Work out the finished part from the listing and answer in its coordinate system (mm). Face numbers are marked on the shaded views. Give positions to 0.01 mm unless a question says otherwise; leave off trailing zeros. Write each loop counter-clockwise with the first axis right and the second up, starting at its lowest first coordinate (ties: lowest second). Pieces come first, ordered by that corner, then holes. Notation, with made-up numbers: (18.5, -11.5) -> (30.5, -11.5) arc R20 ccw to (30.5, 26.5) -> close; hole circle Ø4 at (34.25, 88). An arc over 180 degrees is marked (long way). Use a Markdown table: item, result. Add a question column.
Q1. For a pull along X with two mould halves and no side action, classify the marked faces 1, 2, 3 and 4 as pulls with the +X half, pulls with the -X half, needs draft (parallel to the pull), parting line crosses it, or undercut.
Q2. Section B-B, the plane x = -8 is taken. Give the vertices of the cut face in (y, z).
Q3. Consider line 1 (Z direction, x = -15.5, y = -14.5); line 2 (Z direction, x = 14, y = -6); line 3 (X direction, y = -5.25, z = -12.5). Determine where each line is inside the solid, lowest interval first.
Q4. Section C-C, the plane z = 7 is taken. Give the vertices of the cut face in (x, y), plus the area to 3 significant figures.
Q5. Each of these flat-tipped pins is pushed along its axis until it touches: pin 1 Ø5 at (x, y) = (-0.5, -10) entering from -Z; pin 2 Ø6 at (x, y) = (-16, -16.5) entering from -Z; pin 3 Ø1.5 at (y, z) = (-12, 5) entering from -X; pin 4 Ø8 at (x, y) = (12.5, -13) entering from +Z. Where does it stop, or does it pass through?
Q6. Section A-A, the plane x = -17 is taken. Give the vertices of the cut face in (y, z).
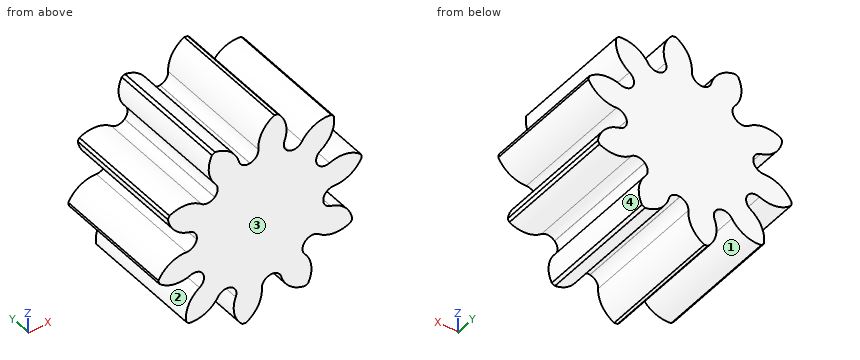
from build123d import *

# Parameters (mm, degrees)
F1_DEPTH = 25


with BuildPart() as f1:
    # F0 (on Front) → F1 (new body)
    with BuildSketch(Plane.XZ):
        with BuildLine():
            ThreePointArc((-0.348561, 15.07019), (-0.783748, 13.691524), (-2.03445, 12.966366))
            ThreePointArc((-2.03445, 12.966366), (-2.044108, 12.964847), (-2.053766, 12.96332))
            ThreePointArc((-2.053766, 12.96332), (-2.063307, 12.961805), (-2.072847, 12.960283))
            ThreePointArc((-2.072847, 12.960283), (-3.48649, 13.263394), (-4.326471, 14.440126))
            ThreePointArc((-4.326471, 14.440126), (-6.102339, 17.389838), (-9.209645, 18.872796))
            ThreePointArc((-9.209645, 18.872796), (-9.534613, 18.710723), (-9.856731, 18.543054))
            ThreePointArc((-9.856731, 18.543054), (-10.48276, 15.157493), (-9.140028, 11.987161))
            ThreePointArc((-9.140028, 11.987161), (-8.681741, 10.616), (-9.267343, 9.294191))
            ThreePointArc((-9.267343, 9.294191), (-9.274264, 9.287285), (-9.28118, 9.280373))
            ThreePointArc((-9.28118, 9.280373), (-9.288008, 9.273539), (-9.294832, 9.2667))
            ThreePointArc((-9.294832, 9.2667), (-10.616657, 8.681004), (-11.987881, 9.139271))
            ThreePointArc((-11.987881, 9.139271), (-15.158386, 10.48181), (-18.54391, 9.85512))
            ThreePointArc((-18.54391, 9.85512), (-18.711551, 9.532987), (-18.873597, 9.208005))
            ThreePointArc((-18.873597, 9.208005), (-17.390082, 6.101058), (-14.440314, 4.325444))
            ThreePointArc((-14.440314, 4.325444), (-13.263604, 3.485525), (-12.960426, 2.071951))
            ThreePointArc((-12.960426, 2.071951), (-12.961966, 2.062295), (-12.963499, 2.052639))
            ThreePointArc((-12.963499, 2.052639), (-12.965006, 2.043097), (-12.966506, 2.033553))
            ThreePointArc((-12.966506, 2.033553), (-13.691622, 0.782765), (-15.070328, 0.347526))
            ThreePointArc((-15.070328, 0.347526), (-18.424445, -0.429914), (-20.795033, -2.926878))
            ThreePointArc((-20.795033, -2.926878), (-20.741312, -3.286025), (-20.68139, -3.64419))
            ThreePointArc((-20.68139, -3.64419), (-17.654983, -5.285774), (-14.224891, -4.988446))
            ThreePointArc((-14.224891, -4.988446), (-12.779221, -4.976302), (-11.703067, -5.941704))
            ThreePointArc((-11.703067, -5.941704), (-11.698638, -5.95042), (-11.694202, -5.959133))
            ThreePointArc((-11.694202, -5.959133), (-11.689812, -5.96774), (-11.685416, -5.976342))
            ThreePointArc((-11.685416, -5.976342), (-11.536853, -7.414464), (-12.396423, -8.576962))
            ThreePointArc((-12.396423, -8.576962), (-14.652992, -11.177425), (-15.103159, -14.590907))
            ThreePointArc((-15.103159, -14.590907), (-14.848597, -14.849888), (-14.589595, -15.104427))
            ThreePointArc((-14.589595, -15.104427), (-11.176282, -14.65362), (-8.576044, -12.396919))
            ThreePointArc((-8.576044, -12.396919), (-7.41361, -11.537351), (-5.975534, -11.68583))
            ThreePointArc((-5.975534, -11.68583), (-5.966827, -11.690278), (-5.958117, -11.69472))
            ThreePointArc((-5.958117, -11.69472), (-5.949507, -11.699102), (-5.940895, -11.703478))
            ThreePointArc((-5.940895, -11.703478), (-4.975398, -12.779619), (-4.987505, -14.225343))
            ThreePointArc((-4.987505, -14.225343), (-5.284594, -17.65554), (-3.642392, -20.681706))
            ThreePointArc((-3.642392, -20.681706), (-3.284223, -20.741598), (-2.925071, -20.795287))
            ThreePointArc((-2.925071, -20.795287), (-0.42862, -18.424281), (0.348561, -15.07019))
            ThreePointArc((0.348561, -15.07019), (0.783748, -13.691524), (2.03445, -12.966366))
            ThreePointArc((2.03445, -12.966366), (2.044108, -12.964847), (2.053766, -12.96332))
            ThreePointArc((2.053766, -12.96332), (2.063307, -12.961805), (2.072847, -12.960283))
            ThreePointArc((2.072847, -12.960283), (3.48649, -13.263394), (4.326471, -14.440126))
            ThreePointArc((4.326471, -14.440126), (6.102339, -17.389838), (9.209645, -18.872796))
            ThreePointArc((9.209645, -18.872796), (9.534613, -18.710723), (9.856731, -18.543054))
            ThreePointArc((9.856731, -18.543054), (10.48276, -15.157493), (9.140028, -11.987161))
            ThreePointArc((9.140028, -11.987161), (8.681741, -10.616), (9.267343, -9.294191))
            ThreePointArc((9.267343, -9.294191), (9.274264, -9.287285), (9.28118, -9.280373))
            ThreePointArc((9.28118, -9.280373), (9.288008, -9.273539), (9.294832, -9.2667))
            ThreePointArc((9.294832, -9.2667), (10.616657, -8.681004), (11.987881, -9.139271))
            ThreePointArc((11.987881, -9.139271), (15.158386, -10.48181), (18.54391, -9.85512))
            ThreePointArc((18.54391, -9.85512), (18.711551, -9.532987), (18.873597, -9.208005))
            ThreePointArc((18.873597, -9.208005), (17.390082, -6.101058), (14.440314, -4.325444))
            ThreePointArc((14.440314, -4.325444), (13.263604, -3.485525), (12.960426, -2.071951))
            ThreePointArc((12.960426, -2.071951), (12.961966, -2.062295), (12.963499, -2.052639))
            ThreePointArc((12.963499, -2.052639), (12.965006, -2.043097), (12.966506, -2.033553))
            ThreePointArc((12.966506, -2.033553), (13.691622, -0.782765), (15.070328, -0.347526))
            ThreePointArc((15.070328, -0.347526), (18.424445, 0.429914), (20.795033, 2.926878))
            ThreePointArc((20.795033, 2.926878), (20.741312, 3.286025), (20.68139, 3.64419))
            ThreePointArc((20.68139, 3.64419), (17.654983, 5.285774), (14.224891, 4.988446))
            ThreePointArc((14.224891, 4.988446), (12.779221, 4.976302), (11.703067, 5.941704))
            ThreePointArc((11.703067, 5.941704), (11.698638, 5.95042), (11.694202, 5.959133))
            ThreePointArc((11.694202, 5.959133), (11.689812, 5.96774), (11.685416, 5.976342))
            ThreePointArc((11.685416, 5.976342), (11.536853, 7.414464), (12.396423, 8.576962))
            ThreePointArc((12.396423, 8.576962), (14.652992, 11.177425), (15.103159, 14.590907))
            ThreePointArc((15.103159, 14.590907), (14.848597, 14.849888), (14.589595, 15.104427))
            ThreePointArc((14.589595, 15.104427), (11.176282, 14.65362), (8.576044, 12.396919))
            ThreePointArc((8.576044, 12.396919), (7.41361, 11.537351), (5.975534, 11.68583))
            ThreePointArc((5.975534, 11.68583), (5.966827, 11.690278), (5.958117, 11.69472))
            ThreePointArc((5.958117, 11.69472), (5.949507, 11.699102), (5.940895, 11.703478))
            ThreePointArc((5.940895, 11.703478), (4.975398, 12.779619), (4.987505, 14.225343))
            ThreePointArc((4.987505, 14.225343), (5.284594, 17.65554), (3.642392, 20.681706))
            ThreePointArc((3.642392, 20.681706), (3.284223, 20.741598), (2.925071, 20.795287))
            ThreePointArc((2.925071, 20.795287), (0.42862, 18.424281), (-0.348561, 15.07019))
        make_face()
    extrude(amount=F1_DEPTH)


solid = f1.part
Result set:
| question | item | result |
|---|---|---|
| 1 | face 1 | undercut |
| 1 | face 2 | pulls with the -X half |
| 1 | face 3 | needs draft |
| 1 | face 4 | pulls with the +X half |
| 2 | outline | (-25, -11.81) -> (0, -11.81) -> (0, 18.55) -> (-25, 18.55) -> close |
| 3 | line 1 | z = -5.34 to 0.36, 4.71 to 10.51 |
| 3 | line 2 | z = -10.24 to -4.16, -0.58 to 4.91, 10.07 to 15.17 |
| 3 | line 3 | x = -15.07 to -8.64, -5.11 to 9.52 |
| 4 | outline | (-18.06, -25) -> (11.47, -25) -> (11.47, 0) -> (-18.06, 0) -> close |
| 4 | area | 738 mm2 |
| 5 | pin 1 | stops at z = -20.8 |
| 5 | pin 2 | stops at z = -15.18 |
| 5 | pin 3 | stops at x = -17.04 |
| 5 | pin 4 | stops at z = 15.18 |
| 6 | outline | (-25, -5.38) -> (0, -5.38) -> (0, 0.16) -> (-25, 0.16) -> close; (-25, 5.71) -> (0, 5.71) -> (0, 10.4) -> (-25, 10.4) -> close |
